```python
from build123d import *

# Parameters (mm, degrees)
BOSS_EXTRUDE1_DEPTH = 50
SKETCH3_R           = 42.5
SKETCH3_R_2         = 16
BOSS_EXTRUDE2_DEPTH = 5
SKETCH4_R           = 16
CUT_EXTRUDE1_DEPTH  = 26
SKETCH6_W           = 100.044775272
SKETCH6_H           = 92
CUT_EXTRUDE3_DEPTH  = 2
FILLET1_R           = 3


with BuildPart() as part:
    # Sketch2 → Boss-Extrude1 (new body, symmetric)
    with BuildSketch(Plane.XY):
        Polygon((0, 0), (0, 25), (-100, 25), (-100, 18), (-32.823085464, 0), align=None)
    extrude(amount=BOSS_EXTRUDE1_DEPTH, both=True)

    # Sketch3 → Boss-Extrude2 (add)
    with BuildSketch(Plane(origin=(0, 25, 0), x_dir=(1, 0, 0), z_dir=(0, 1, 0))):
        with Locations((-50, 0)):
            Circle(SKETCH3_R)
        with Locations((-50, 0)):
            Circle(SKETCH3_R_2, mode=Mode.SUBTRACT)
    extrude(amount=BOSS_EXTRUDE2_DEPTH)

    # Sketch4 → Cut-Extrude1 (cut, through all)
    with BuildSketch(Plane(origin=(0, 25, 0), x_dir=(1, 0, 0), z_dir=(0, 1, 0))):
        with Locations((-50, 0)):
            Circle(SKETCH4_R)
    extrude(amount=-CUT_EXTRUDE1_DEPTH, mode=Mode.SUBTRACT)

    # Sketch6 → Cut-Extrude3 (cut)
    with BuildSketch(Plane(origin=(-2.198729811, -8.205771366, 0), x_dir=(0.965925826, -0.258819045, 0), z_dir=(-0.258819045, -0.965925826, 0))):
        with Locations((-62.936330428, 0)):
            Rectangle(SKETCH6_W, SKETCH6_H)
    extrude(amount=-CUT_EXTRUDE3_DEPTH, mode=Mode.SUBTRACT)

    # Fillet1
    fillet1_edges = [part.edges().sort_by_distance(p)[0] for p in [
        (-50, 25, 50),
        (-100, 21.5, 50),
        (-92.5, 25, 0),
        (-66.411542732, 9, 50),
        (-16.411542732, 0, 50),
        (-66.411542732, 9, -50),
        (-100, 21.5, -50),
        (-50, 25, -50),
        (0, 12.5, -50),
        (-16.411542732, 0, -50),
        (0, 12.5, 50),
        (-100, 25, 0),
        (0, 25, 0),
        (0, 0, 0),
    ]]
    fillet(fillet1_edges, radius=FILLET1_R)


solid = part.part
```
Check sheet for the modelled part. Datum: model origin and axes. Units: mm. A direction names the side the tool comes from. Round coordinates to 2 decimals unless told otherwise and drop trailing zeros. Loops run counter-clockwise (first coordinate to the right, second up) from the corner with the lowest first, then second, coordinate; pieces in that order, holes last. Notation, with made-up numbers: (54.25, 14) - (84.25, 14) arc R10 cw to (84.25, 27) - close; hole circle Ø1 at (70.25, 60). An arc over 180 degrees is marked (long way). Write item = value, one per line. Start each with the question number.
Q1. Access from +Z, -Z, +X, -X, +Y, -Y to the whole of each face (thin tool, end or side, straight path). Record for faces 4 (the face through (-63, 9, -46)), 5 (the face through (-40, 15, 50)), 6 (the face through (-92.46, 28.99, -1.87)).
Q2. Thickness scan on L1, parallel to Z at x = -50, y = 10; L2, parallel to X at y = 28, z = 0; L3, parallel to Y at x = -23.5, z = 42. Record the ranges inside material, lowest first.
Q3. Section check B-B (y = 23.5). Record the boundary of the cut face in (x, z), plus the area to 3 significant figures.
Q4. Section check A-A (z = 0). Record the boundary of the cut face in (x, y), plus the area to 3 significant figures.
Q5. Release check for a two-part mould opening along Z. For faces 1 (the face through (-71.395, 12.406, 0.644)), 2 (the face through (-51, 30, 18)), 3 (the face through (-0.86, 12.63, -49.1)) record: pulls with the +Z half, pulls with the -Z half, needs draft (parallel to the pull), parting line crosses it, or undercut.
Derived:
q1.face_4 = -X, -Y
q1.face_5 = +Z, +X, -X, +Y, -Y
q1.face_6 = +Y
q2.L1 = -50 to -16, 16 to 50
q2.L2 = -92.5 to -66, -34 to -7.5
q2.L3 = 0 to 25
q3.outline = (-99.6, -47) arc R2.6 ccw to (-97, -49.6) - (-3, -49.6) arc R2.6 ccw to (-0.4, -47) - (-0.4, 47) arc R2.6 ccw to (-3, 49.6) - (-97, 49.6) arc R2.6 ccw to (-99.6, 47) - close; hole circle Ø32 at (-50, 0)
q3.area = 9,030 mm^2
q4.outline = (-100, 20.07) - (-66, 10.96) - (-66, 30) - (-92.5, 30) - (-92.5, 28) arc R3 cw to (-95.5, 25) - (-97, 25) arc R3 ccw to (-100, 22) - close; (-34, 2.39) - (-25.1, 0) - (-3, 0) arc R3 ccw to (0, 3) - (0, 22) arc R3 ccw to (-3, 25) - (-4.5, 25) arc R3 cw to (-7.5, 28) - (-7.5, 30) - (-34, 30) - close
q4.area = 1,420 mm^2
q5.face_1 = undercut
q5.face_2 = needs draft
q5.face_3 = pulls with the -Z half
